Autodesk Inventor part; units mm, degrees
ref_plane "YZ Plane" through (0, 0, 0) normal (1, 0, 0) x (0, 1, 0)
ref_plane "XZ Plane" through (0, 0, 0) normal (0, 1, 0) x (-1, 0, 0)
ref_plane "XY Plane" through (0, 0, 0) normal (0, 0, 1) x (1, 0, 0)
sketch "Sketch1" plane through (0, 0, 0) normal (0, 0, 1) x (1, 0, 0)
  line L0 (0, 0) -> (542, 0)
  line L1 (0, 0) -> (0, 38)
  line L2 (0, 38) -> (512.3111, 38)
  line L3 (542, 0) -> (512.3111, 38)
  dimension "d0" = 542
  dimension "d1" = 38
  dimension "d2" = 52
extrude "Extrusion1" add sketch "Sketch1" along normal blind 114
sketch "Sketch3" plane through (0, 0, 0) normal (0, -1, 0) x (1, 0, 0)
  line L0 (0, 0) -> (0, 114)
  circle A0 centre (38, 57) radius 7.5
  dimension "d21" = 38
  dimension "d22" = 15
extrude "Extrusion2" cut sketch "Sketch3" against normal blind 1
properties part number "2p3s37" material "Wood (Cherry)"
CAD build for the part. Positions are in the model's coordinates, mm. A direction names the side the tool comes from. Coordinates: 2 decimals unless noted, no trailing zeros. Order: outer loops, then holes, each group sorted by start corner. A loop starts at its lowest first (then second) coordinate and runs counter-clockwise, first axis right, second up.
Item 1: Band-saw the part on B-B on y = 32. List the corners of the cut face in (x, z).
Check sheet entries:
outline: (0, 0) - (517, 0) - (517, 114) - (0, 114) - close
Item 2: Drill centre lines: L1, parallel to Z at x = 38, y = 0.3; L2, parallel to X at y = 7.5, z = 51.5; L3, parallel to X at y = 5.5, z = 31.5. Where is each one in solid material? Low to high.
Check sheet entries:
L1: z = 0 to 49.5, 64.5 to 114
L2: x = 0 to 536.14
L3: x = 0 to 537.7
Item 3: Band-saw the part on C-C on z = 97. List the corners of the cut face in (x, y), plus the area to 3 significant figures.
Check sheet entries:
outline: (0, 0) - (542, 0) - (512.31, 38) - (0, 38) - close
area: 20,000 mm2
Item 4: 3-axis set-ups, long thin cutter, end or side, ignore diameter. For faces 1 (the face through (0, 19, 56)), 2 (the face through (37.024, 0.493, 64.436)): which of +Z, -Z, +X, -X, +Y, -Y reach the whole face in a straight line?
Check sheet entries:
face 1: +Z, -Z, -X, +Y, -Y
face 2: -Y
Item 5: Two-plate mould, pull along Z, no slides. Class faces 3 (the face through (527.363, 18.734, 56.202)), 4 (the face through (267, 19, 114)), 5 (the face through (38, 1, 57)): +Z half, -Z half, draft (parallel to the pull), parting line (faces both ways), or undercut.
Check sheet entries:
face 3: draft
face 4: +Z half
face 5: undercut
Item 6: Pin check, flat tips, straight feed: pin 1 Ø13.5 at (x, z) = (38, 57) entering from -Y; pin 2 Ø3 at (y, z) = (29, 55) entering from +X. Stop position of each tip, or through.
Check sheet entries:
pin 1: stops at y = 1
pin 2: stops at x = 520.51
Item 7: Band-saw the part on A-A on z = 57. List the corners of the cut face in (x, y), plus the area to 3 significant figures.
Check sheet entries:
outline: (0, 0) - (30.5, 0) - (30.5, 1) - (45.5, 1) - (45.5, 0) - (542, 0) - (512.31, 38) - (0, 38) - close
area: 20,000 mm2
